Here's how the part is built. I have some questions about the finished solid (model axes, mm). A direction names the side the tool comes from. Round coordinates to 2 decimals unless told otherwise and drop trailing zeros. Write each loop counter-clockwise with the first axis right and the second up, starting at its lowest first coordinate (ties: lowest second). Pieces come first, ordered by that corner, then holes. Notation, with made-up numbers: M -14,-26 L 36,-26 A37 cw 36,10 Z; hole C 21,49 d4. An arc over 180 degrees is marked long. Write item = value, one per line. Start each with the question number.
(1) I want a section at A-A (z = 12). List the corners of the cut face in (x, y) for me, and give its area (3 significant figures).
(2) I want a section at D-D (z = 6). List the corners of the cut face in (x, y) for me, and give its area (3 significant figures).
(3) If we mould it in two halves opening along Z, with no side actions, what happens to faces 3 (the flat face through (5, 19, 30)), 4 (the cylindrical face through (5, 20, 19)), 5 (the flat face through (20, 20, 15))? For each: released by +Z, released by -Z, zero draft, split by the parting line, or undercut.
(4) I need wall thicknesses on line 1 along Z through (x, y) = (5, 20.35); line 2 along X through (y, z) = (19.2, 12); line 3 along Y through (x, z) = (9.5, 19.5). Which ranges of each line are inside material? Lowest first, please.
(5) Will these pins go through, and if not, where does the flat tip stop? pin 1 Ø9 at (x, z) = (12.5, 12) entering from -Y; pin 2 Ø5.5 at (y, z) = (11.5, 19) entering from +X.
(6) I want a section at B-B (x = 5). List the corners of the cut face in (y, z) for me.
(7) On a 3-axis mill with a long thin cutter (end or side, diameter ignored), from which of +Z, -Z, +X, -X, +Y, -Y can I reach the whole of each face in a straight line? I mean faces 1 (the cylindrical face through (5, 20, 11)), 2 (the flat face through (11, 18.5, 15)). Say none if no direction works.
(8) I want a section at C-C (y = 13.5). List the corners of the cut face in (x, z) for me, and give its area (3 significant figures).
```python
from build123d import *

# Parameters (mm, degrees)
BOSS_EXTRUDE1_DEPTH             = 30
F_2_0MM_CLEARANCE_DOWEL_HOLE1_D = 2


with BuildPart() as part:
    # Sketch1 → Boss-Extrude1 (new body)
    with BuildSketch(Plane.XY):
        with BuildLine():
            Line((0, 19), (0, 0))
            Line((0, 0), (1.5, 0))
            Line((1.5, 0), (1.5, 18.5))
            Line((1.5, 18.5), (20, 18.5))
            Line((20, 18.5), (20, 20))
            Line((20, 20), (1, 20))
            ThreePointArc((1, 20), (0.292893219, 19.707106781), (0, 19))
        make_face()
        with BuildLine():
            Line((-1.5, 0), (0, 0))
            Line((0, 0), (0, 19))
            ThreePointArc((0, 19), (0.292893219, 19.707106781), (1, 20))
            Line((1, 20), (20, 20))
            Line((20, 20), (20, 21.5))
            Line((20, 21.5), (1, 21.5))
            ThreePointArc((1, 21.5), (-0.767766953, 20.767766953), (-1.5, 19))
            Line((-1.5, 19), (-1.5, 0))
        make_face()
    extrude(amount=BOSS_EXTRUDE1_DEPTH)

    # Ø2.0mm Clearance Dowel Hole1 (through all)
    with Locations(Plane(origin=(-21.929397557, 18.5, -58.5), x_dir=(-1, 0, 0), z_dir=(0, -1, 0))):
        with Locations((-26.929397557, -76.5), (-26.929397557, -70.5)):
            Hole(F_2_0MM_CLEARANCE_DOWEL_HOLE1_D / 2)


solid = part.part
```
Returned:
q1.outline = M -1.5,0 L 1.5,0 L 1.5,18.5 L 4,18.5 L 4,21.5 L 1,21.5 A2.5 ccw -1.5,19 Z; M 6,18.5 L 20,18.5 L 20,21.5 L 6,21.5 Z
q1.area = 113 mm²
q2.outline = M -1.5,0 L 1.5,0 L 1.5,18.5 L 20,18.5 L 20,21.5 L 1,21.5 A2.5 ccw -1.5,19 Z
q2.area = 119 mm²
q3.face_3 = released by +Z
q3.face_4 = undercut
q3.face_5 = zero draft
q4.line_1 = 0 to 11, 13 to 17, 19 to 30
q4.line_2 = -1.49 to 4, 6 to 20
q4.line_3 = 18.5 to 21.5
q5.pin_1 = 18.5
q5.pin_2 = 1.5
q6.outline = M 18.5,0 L 21.5,0 L 21.5,11 L 18.5,11 Z; M 18.5,13 L 21.5,13 L 21.5,17 L 18.5,17 Z; M 18.5,19 L 21.5,19 L 21.5,30 L 18.5,30 Z
q7.face_1 = +Y, -Y
q7.face_2 = +Z, -Z, +X, -Y
q8.outline = M -1.5,0 L 1.5,0 L 1.5,30 L -1.5,30 Z
q8.area = 90.0 mm²
